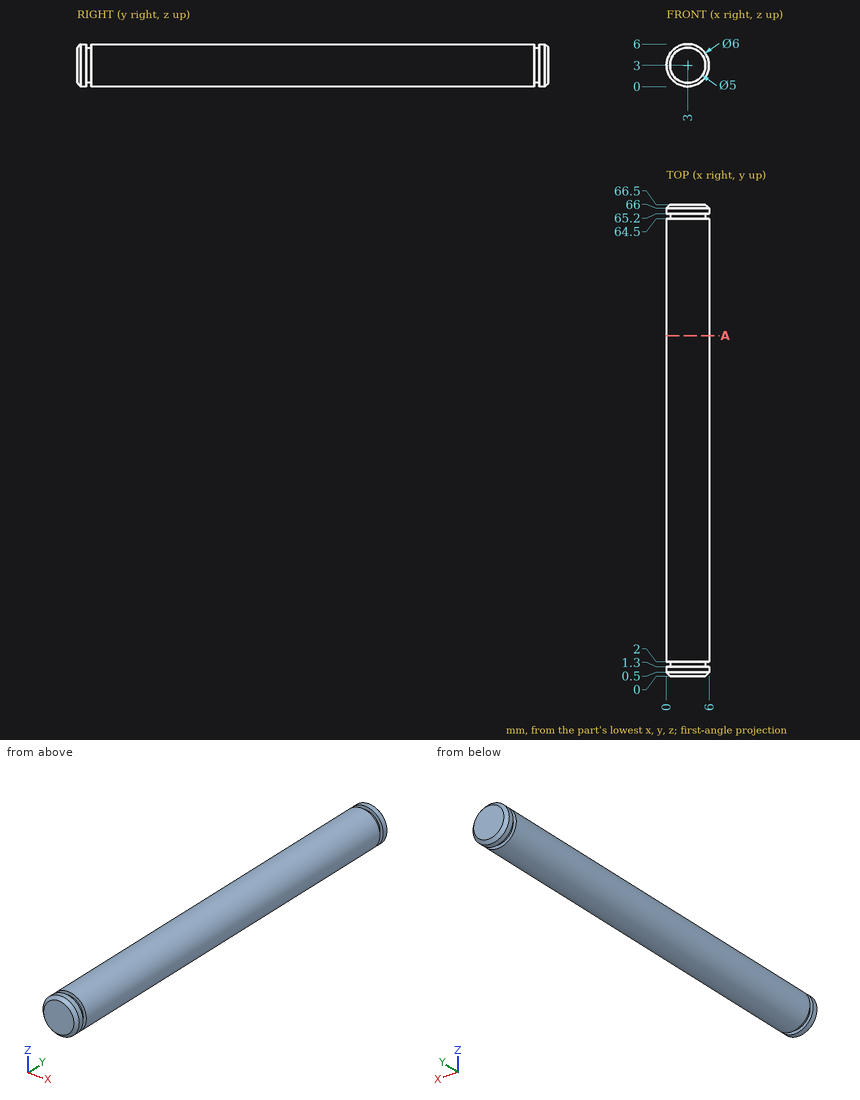
Here's the drawing with two shaded views (mm, measured from the low corner). I have some questions. Coordinates: 2 decimals unless noted, no trailing zeros. Order: outer loops, then holes, each group sorted by start corner. A loop starts at its lowest first (then second) coordinate and runs counter-clockwise, first axis right, second up. Notation, with made-up numbers: (89.25, 82.25) - (127.25, 82.25) arc R17 cw to (127.25, 111.25) - close; hole circle Ø5 at (36.5, 71.25). An arc over 180 degrees is marked (long way). Use CSV: the item, a comma, the result in double quotes. Start each with the question number.
1. Suppose I cut it at A-A on y = 48. List the corners of the cut face in (x, z) for me.
2. I'm going to push flat-ended pins straight in: pin 1 (1 mm diameter, centred on y = 15.5, z = 4, fed in from +X); pin 2 (2 mm diameter, centred on y = 40.5, z = 1, fed in from +X); pin 3 (1.8 mm diameter, centred on x = 4.5, z = 4.5, fed in from -Y). Where does each tip first touch, or does it pass through?
3. Please list where these lines run through material, in increasing order: line 1 (Y direction, x = 0.6, z = 1.75); line 2 (Y direction, x = 2, z = 0.65); line 3 (X direction, y = 43, z = 2.9). Write a range as from..to.
Output:
1,outline,"circle Ø6 at (3, 3)"
2,pin 1,"stops at x = 5.96"
2,pin 2,"stops at x = 5.83"
2,pin 3,"stops at y = 0"
3,line 1,"y = 0.21..1.3, 2..64.5, 65.2..66.29"
3,line 2,"y = 0.05..1.3, 2..64.5, 65.2..66.45"
3,line 3,"x = 0..6"
